```python
from build123d import *

# Parameters (mm, degrees)
F0_R     = 8.047855898
F0_R_2   = 1.0743657774
F1_DEPTH = 25


# Not quite as in the source:
# - the program builds the solid bodies; features that only make, move or delete a surface that nothing else refers to are left out


with BuildPart() as f1:
    # F0 (on Front) → F1 (new body)
    with BuildSketch(Plane.XZ):
        Polygon((75, 46.0328937352), (75, 107.7262044382), (-75, 107.7262044382), (-75, 46.0328937352), (-75, -36.6851300407), (-75, -92.2737955618), (75, -92.2737955618), (75, -36.6851300407), align=None)
        with Locations((0, -35.9561647287)):
            Circle(F0_R, mode=Mode.SUBTRACT)
        Polygon((44.7407775558, -21.2889015805), (-30.3720422538, -21.2889015805), (-41.1018976561, -10.5590461782), (-30.3720422538, 0.1708092241), (44.7407775558, 0.1708092241), (55.4706329581, -10.5590461782), align=None, mode=Mode.SUBTRACT)
        with Locations((-48.4804458196, 44.5564172655)):
            Circle(F0_R_2, mode=Mode.SUBTRACT)
        with Locations((-44.1829827099, 44.5564172655)):
            Circle(F0_R_2, mode=Mode.SUBTRACT)
        with Locations((-39.8855196001, 44.5564172655)):
            Circle(F0_R_2, mode=Mode.SUBTRACT)
        with Locations((-49.0825107104, 65.3187614809)):
            Circle(F0_R_2, mode=Mode.SUBTRACT)
        with Locations((-44.7850476006, 65.3187614809)):
            Circle(F0_R_2, mode=Mode.SUBTRACT)
        with Locations((-40.4875844908, 65.3187614809)):
            Circle(F0_R_2, mode=Mode.SUBTRACT)
        with Locations((40.4036690891, 46.6322604282)):
            Circle(F0_R_2, mode=Mode.SUBTRACT)
        with Locations((44.7011321989, 46.6322604282)):
            Circle(F0_R_2, mode=Mode.SUBTRACT)
        with Locations((48.9985953086, 46.6322604282)):
            Circle(F0_R_2, mode=Mode.SUBTRACT)
        with Locations((40.4036690891, 63.9077951499)):
            Circle(F0_R_2, mode=Mode.SUBTRACT)
        with Locations((44.7011321989, 63.9077951499)):
            Circle(F0_R_2, mode=Mode.SUBTRACT)
        with Locations((48.9985953086, 63.9077951499)):
            Circle(F0_R_2, mode=Mode.SUBTRACT)
        with BuildLine():
            add(Edge.make_bspline(
                [(75, 46.0328937352), (91.3344780181, 49.9824236443), (133.3315352118, 60.1369344463), (97.1245297955, 0.0384474003), (75, -36.6851300407)],
                knots=[0, 0, 0, 0, 0.3889433953, 1, 1, 1, 1], degree=3))
            Line((75, 46.0328937352), (75, -36.6851300407))
        make_face()
        with BuildLine():
            Line((-75, -36.6851300407), (-75, 46.0328937352))
            add(Edge.make_bspline(
                [(-75, 46.0328937352), (-91.3344780181, 49.9824236443), (-133.3315352118, 60.1369344463), (-97.1245297955, 0.0384474003), (-75, -36.6851300407)],
                knots=[0, 0, 0, 0, 0.3889433953, 1, 1, 1, 1], degree=3))
        make_face()
    extrude(amount=F1_DEPTH)


solid = f1.part
```
The model under review builds one solid part; all positions refer to its coordinate system, in mm. A direction names the side the tool comes from. Give positions to 0.01 mm unless a question says otherwise; leave off trailing zeros. Write each loop counter-clockwise with the first axis right and the second up, starting at its lowest first coordinate (ties: lowest second). Pieces come first, ordered by that corner, then holes. Notation, with made-up numbers: (-13.5, 30.25) - (9.5, 30.25) arc R21 cw to (9.5, 46.25) - close; hole circle Ø2 at (7, -30.5). An arc over 180 degrees is marked (long way). Answer in a Markdown table with one row per item. Add a question column.
1. We need section A-A on x = 0. Write out the cut boundary in (y, z).
2. Draft analysis for pull direction X (two halves, no side actions). For faces 1 (the flat face through (-1, -12, -92.274)), 2 (the flat face through (-35.812, -12.325, -5.269)), 3 (the flat face through (-75, -12, -64)), state which applies: +X half, -X half, draft (parallel to the pull), parting line (faces both ways), or undercut.
3. Insertion check: P1, Ø1, axis at y = -6, z = -15.5, coming from the +X side; P2, Ø12.5, axis at y = -10.5, z = -64.5, coming from the -X side; P3, Ø12, axis at x = 83.5, y = -14.5, coming from the +Z side; P4, Ø1.7, axis at x = 44.7, z = 46.63, coming from the -Y side. Each pin has a flat end and moves straight along its axis. Give the tip position at first contact, or say it passes through.
4. We need section B-B on z = -63. Write out the cut boundary in (x, y).
5. Wall thickness on line 1 along Z through (x, y) = (0, -12.25); line 2 along Z through (x, y) = (-18.5, -8.75); line 3 along X through (y, z) = (-23.75, 86): over which ranges is each line inside the solid? List them lowest first. Write a range as [from, to].
6. Tool access review of faces 4 (the flat face through (50.03, -12.32, -5.12)), 5 (the flat face through (75, -12, -65)), 6 (the flat face through (-2, 0, 9)): name each direction out of +Z, -Z, +X, -X, +Y, -Y from which nothing blocks a thin tool from reaching the whole face with its end or side.
7. We need section C-C on y = -16.5. State how many separate pieces and enclosed holes the cut face has, then the cut area to 3 significant figures.
Ans:
| question | item | result |
|---|---|---|
| 1 | outline | (-25, -92.27) - (0, -92.27) - (0, -44) - (-25, -44) - close; (-25, -27.91) - (0, -27.91) - (0, -21.29) - (-25, -21.29) - close; (-25, 0.17) - (0, 0.17) - (0, 107.73) - (-25, 107.73) - close |
| 2 | face 1 | draft |
| 2 | face 2 | undercut |
| 2 | face 3 | -X half |
| 3 | P1 | stops at x = 87.96 |
| 3 | P2 | stops at x = -75 |
| 3 | P3 | stops at z = 49.32 |
| 3 | P4 | passes through |
| 4 | outline | (-75, -25) - (75, -25) - (75, 0) - (-75, 0) - close |
| 5 | line 1 | z = [-92.27, -44], [-27.91, -21.29], [0.17, 107.73] |
| 5 | line 2 | z = [-92.27, -21.29], [0.17, 107.73] |
| 5 | line 3 | x = [-75, 75] |
| 6 | face 4 | +Y, -Y |
| 6 | face 5 | -Z, +X, +Y, -Y |
| 6 | face 6 | +Z, -Z, +X, -X, +Y |
| 7 | separate pieces | 1 |
| 7 | enclosed holes | 14 |
| 7 | area | 31,900 mm^2 |
